```python
from build123d import *

# Parameters (mm, degrees)
F0_W     = 139.7
F0_H     = 91.44
F1_DEPTH = 19.05
F2_W     = 125.73
F2_H     = 6.35
F3_DEPTH = 25.4
F4_W     = 16.51
F4_H     = 88.9
F5_DEPTH = 12.7
F6_W     = 16.51
F6_H     = 82.55
F7_DEPTH = 125.73


with BuildPart() as f1:
    # F0 (on Right) → F1 (new body)
    with BuildSketch(Plane.YZ):
        Rectangle(F0_W, F0_H)
    extrude(amount=F1_DEPTH)

    # F2 (on face) → F3 (cut)
    with BuildSketch(Plane.YZ.offset(19.05)):
        with Locations((-6.985, -42.545)):
            Rectangle(F2_W, F2_H)
    extrude(amount=-F3_DEPTH, mode=Mode.SUBTRACT)

    # F4 (on face) → F5 (cut)
    with BuildSketch(Plane(origin=(0, 69.85, 0), x_dir=(-1, 0, 0), z_dir=(0, 1, 0))):
        with Locations((-9.525, 0)):
            Rectangle(F4_W, F4_H)
    extrude(amount=-F5_DEPTH, mode=Mode.SUBTRACT)

    # F6 (on face) → F7 (cut)
    with BuildSketch(Plane(origin=(0, 57.15, 0), x_dir=(-1, 0, 0), z_dir=(0, 1, 0))):
        with Locations((-9.525, 3.175)):
            Rectangle(F6_W, F6_H)
    extrude(amount=-F7_DEPTH, mode=Mode.SUBTRACT)


solid = f1.part
```
Check sheet for the modelled part. Datum: model origin and axes. Units: mm. A direction names the side the tool comes from. Round coordinates to 2 decimals unless told otherwise and drop trailing zeros. Write each loop counter-clockwise with the first axis right and the second up, starting at its lowest first coordinate (ties: lowest second). Pieces come first, ordered by that corner, then holes. Notation, with made-up numbers: (6.25, 68) -> (26.25, 68) arc R15 ccw to (26.25, 74) -> close; hole circle Ø6 at (70.5, 37.25). An arc over 180 degrees is marked (long way). Put each result on its own line as item: value.
(1) Go/stop test with flat-tipped pins: pin 1 Ø5 at (x, y) = (3.5, 33) entering from -Z; pin 2 Ø1.9 at (x, z) = (10, -41.5) entering from +Y; pin 3 Ø5 at (x, z) = (5, -43.5) entering from -Y. Record where each tip stops, or that it passes through.
Values found:
pin 1: stops at z = -39.37
pin 2: stops at y = 57.15
pin 3: stops at y = 55.88
(2) Tool access check on faces 1 (the face through (9, 63, -45.72)), 2 (the face through (1.27, 2, -1)), 3 (the face through (10, 55.88, -43)). Record the directions out of +Z, -Z, +X, -X, +Y, -Y that give a thin tool (end or side, any length) a straight path to the whole face; none if there is none.
Values found:
face 1: -Z, +X, -X, +Y, -Y
face 2: +Y
face 3: -Z, +X, -X, -Y
(3) Mould release check, pull along Z, two halves, no side actions. Record for faces 4 (the face through (10, 2, 44.45)), 5 (the face through (10, -8, -39.37)), 6 (the face through (1, 69.85, 0)): released by +Z, released by -Z, zero draft, split by the parting line, or undercut.
Values found:
face 4: undercut
face 5: released by -Z
face 6: zero draft
(4) Sectioned sample at C-C (x = 5). Enter the section's corners in (y, z).
Values found:
outline: (-69.85, -39.37) -> (55.88, -39.37) -> (55.88, -45.72) -> (69.85, -45.72) -> (69.85, -44.45) -> (57.15, -44.45) -> (57.15, -38.1) -> (-68.58, -38.1) -> (-68.58, 44.45) -> (69.85, 44.45) -> (69.85, 45.72) -> (-69.85, 45.72) -> close
(5) Sectioned sample at A-A (y = -36). Enter the section's corners in (x, z), plus the area to 3 significant figures.
Values found:
outline: (0, -39.37) -> (19.05, -39.37) -> (19.05, 45.72) -> (0, 45.72) -> close; hole (1.27, -38.1) -> (17.78, -38.1) -> (17.78, 44.45) -> (1.27, 44.45) -> close
area: 258 mm^2
(6) Sectioned sample at B-B (z = -3). Enter the section's corners in (x, y).
Values found:
outline: (0, -69.85) -> (19.05, -69.85) -> (19.05, 69.85) -> (17.78, 69.85) -> (17.78, -68.58) -> (1.27, -68.58) -> (1.27, 69.85) -> (0, 69.85) -> close
(7) Material ranges on line 1 (X direction, y = -42, z = 32); line 2 (Z direction, x = 6, y = 54.5); line 3 (Z direction, x = 9.25, y = 63), recorded low to high.
Values found:
line 1: x = 0 to 1.27, 17.78 to 19.05
line 2: z = -39.37 to -38.1, 44.45 to 45.72
line 3: z = -45.72 to -44.45, 44.45 to 45.72
